```python
from build123d import *

# Parameters (mm, degrees)
PAD_DEPTH     = 1
SKETCH001_R   = 5.125
SKETCH001_R_2 = 9.9
PAD001_DEPTH  = 1
FILLET_R      = 1


with BuildPart() as part:
    # Sketch → Pad (new body)
    with BuildSketch(Plane.XY):
        with BuildLine():
            Line((70.272578, 45.492899), (78.436266, 3.274963))
            ThreePointArc((46.573742, -8.646925), (67.545071, -16.156101), (78.436266, 3.274963))
            Line((36.055693, 9.509252), (46.573742, -8.646925))
            ThreePointArc((5.490533, 14.509252), (19.215175, 2.485526), (36.055693, 9.509252))
            Line((-5.490533, 14.509252), (5.490533, 14.509252))
            ThreePointArc((-36.055693, 9.509252), (-19.215175, 2.485526), (-5.490533, 14.509252))
            Line((-46.573742, -8.646925), (-36.055693, 9.509252))
            ThreePointArc((-78.436265, 3.274968), (-67.545074, -16.1561), (-46.573742, -8.646925))
            Line((-70.272577, 45.492905), (-78.436265, 3.274968))
            ThreePointArc((-59.5, 62.051362), (-66.503327, 54.824144), (-70.272577, 45.492905))
            Line((-59.5, 62.051362), (-56.5, 72.051362))
            ThreePointArc((-32.5, 72.051362), (-44.5, 76.759252), (-56.5, 72.051362))
            Line((-32.5, 72.051362), (-30.237367, 64.509252))
            Line((-30.237367, 64.509252), (30.237367, 64.509252))
            Line((30.237367, 64.509252), (32.5, 72.051362))
            ThreePointArc((56.5, 72.051362), (44.5, 76.759252), (32.5, 72.051362))
            Line((56.5, 72.051362), (59.5, 62.051362))
            ThreePointArc((70.272578, 45.492899), (66.503328, 54.824142), (59.5, 62.051362))
        make_face()
    extrude(amount=PAD_DEPTH)

    # Sketch001 (on Face20 of Pad) → Pad001 (join)
    with BuildSketch(Plane.XY.offset(1)):
        with BuildLine():
            ThreePointArc((-59.5, 62.051362), (-66.503327, 54.824144), (-70.272577, 45.492905))
            Line((-70.272577, 45.492905), (-78.436265, 3.274968))
            ThreePointArc((-78.436265, 3.274968), (-67.545074, -16.1561), (-46.573742, -8.646925))
            Line((-46.573742, -8.646925), (-36.055693, 9.509252))
            ThreePointArc((-36.055693, 9.509252), (-19.215175, 2.485526), (-5.490533, 14.509252))
            Line((-5.490533, 14.509252), (5.490533, 14.509252))
            ThreePointArc((5.490533, 14.509252), (19.215175, 2.485526), (36.055693, 9.509252))
            Line((36.055693, 9.509252), (46.573742, -8.646925))
            ThreePointArc((46.573742, -8.646925), (67.545071, -16.156101), (78.436266, 3.274963))
            Line((78.436266, 3.274963), (70.272578, 45.492899))
            ThreePointArc((70.272578, 45.492899), (66.503328, 54.824142), (59.5, 62.051362))
            Line((59.5, 62.051362), (56.5, 72.051362))
            ThreePointArc((56.5, 72.051362), (44.5, 76.759252), (32.5, 72.051362))
            Line((32.5, 72.051362), (30.237367, 64.509252))
            Line((30.237367, 64.509252), (-30.237367, 64.509252))
            Line((-30.237367, 64.509252), (-32.5, 72.051362))
            ThreePointArc((-32.5, 72.051362), (-44.5, 76.759252), (-56.5, 72.051362))
            Line((-56.5, 72.051362), (-59.5, 62.051362))
        make_face()
        with BuildLine():
            ThreePointArc((55.140028, 70.584912), (44.5, 74.759252), (33.859972, 70.584912))
            Line((31.437274, 62.509252), (33.859972, 70.584912))
            Line((-31.437274, 62.509252), (31.437274, 62.509252))
            Line((-31.437274, 62.509252), (-33.859972, 70.584912))
            ThreePointArc((-33.859972, 70.584912), (-44.5, 74.759252), (-55.140028, 70.584912))
            Line((-58.357143, 60.410059), (-55.140028, 70.584912))
            ThreePointArc((-58.357143, 60.410059), (-64.826883, 53.733485), (-68.308952, 45.113198))
            Line((-76.47264, 2.895262), (-68.308952, 45.113198))
            ThreePointArc((-76.47264, 2.895262), (-66.844196, -14.282929), (-48.304323, -7.644383))
            Line((-48.304323, -7.644383), (-36.03269, 13.538817))
            ThreePointArc((-36.03269, 13.538817), (-35.306977, 12.060301), (-34.426047, 10.668673))
            ThreePointArc((-34.426047, 10.668673), (-19.538053, 4.459292), (-7.404674, 15.088962))
            ThreePointArc((-7.404674, 15.088962), (-7.209276, 15.794824), (-7.047993, 16.509252))
            Line((-7.047993, 16.509252), (7.047993, 16.509252))
            ThreePointArc((7.047993, 16.509252), (7.209276, 15.794824), (7.404674, 15.088962))
            ThreePointArc((7.404674, 15.088962), (19.538053, 4.459292), (34.426047, 10.668673))
            ThreePointArc((34.426047, 10.668673), (35.306977, 12.060301), (36.03269, 13.538817))
            Line((48.304323, -7.644383), (36.03269, 13.538817))
            ThreePointArc((48.304323, -7.644383), (66.844194, -14.28293), (76.472641, 2.895257))
            Line((76.472641, 2.895257), (68.308953, 45.113193))
            ThreePointArc((68.308953, 45.113193), (64.826884, 53.733483), (58.357143, 60.410059))
            Line((55.140028, 70.584912), (58.357143, 60.410059))
        make_face(mode=Mode.SUBTRACT)
        with Locations((30.375, 40.509252)):
            Circle(SKETCH001_R)
        with Locations((44.5, 54.634252)):
            Circle(SKETCH001_R)
        with Locations((58.625, 40.509252)):
            Circle(SKETCH001_R)
        with Locations((44.5, 26.384252)):
            Circle(SKETCH001_R)
        with Locations((-22, 19.509252)):
            Circle(SKETCH001_R_2)
        with Locations((22, 19.509252)):
            Circle(SKETCH001_R_2)
        Polygon((-58.4, 36.709252), (-51.8, 36.709252), (-49.55, 39.509252), (-49.55, 41.509252), (-51.8, 44.309252), (-58.4, 44.309252), align=None)
        Polygon((-40.7, 26.609252), (-48.3, 26.609252), (-48.3, 33.209252), (-45.5, 35.459252), (-43.5, 35.459252), (-40.7, 33.209252), align=None)
        Polygon((-30.6, 44.309252), (-37.2, 44.309252), (-39.45, 41.509252), (-39.45, 39.509252), (-37.2, 36.709252), (-30.6, 36.709252), align=None)
        Polygon((-48.3, 54.409252), (-40.7, 54.409252), (-40.7, 47.809252), (-43.5, 45.559252), (-45.5, 45.559252), (-48.3, 47.809252), align=None)
    extrude(amount=PAD001_DEPTH)

    # Fillet
    fillet_edges = [part.edges().sort_by_distance(p)[0] for p in [
        (-36.03269, 13.538817, 1.5),
        (-48.3, 26.609252, 1.5),
        (-58.4, 36.709252, 1.5),
        (-58.4, 44.309252, 1.5),
        (-48.3, 54.409252, 1.5),
        (-31.437274, 62.509252, 1.5),
        (-40.7, 54.409252, 1.5),
        (-30.6, 44.309252, 1.5),
        (-30.6, 36.709252, 1.5),
        (-40.7, 26.609252, 1.5),
        (-7.047993, 16.509252, 1.5),
        (36.03269, 13.538817, 1.5),
        (31.437274, 62.509252, 1.5),
        (58.357143, 60.410059, 1.5),
        (7.047993, 16.509252, 1.5),
        (-58.357143, 60.410059, 1.5),
        (-37.2, 36.709252, 1.5),
        (-39.45, 39.509252, 1.5),
        (-43.5, 45.559252, 1.5),
        (-45.5, 45.559252, 1.5),
        (-48.3, 47.809252, 1.5),
        (-51.8, 36.709252, 1.5),
        (-48.3, 33.209252, 1.5),
        (-51.8, 44.309252, 1.5),
        (-49.55, 41.509252, 1.5),
        (-49.55, 39.509252, 1.5),
        (-45.5, 35.459252, 1.5),
        (-43.5, 35.459252, 1.5),
        (-40.7, 33.209252, 1.5),
        (-37.2, 44.309252, 1.5),
        (-40.7, 47.809252, 1.5),
        (-39.45, 41.509252, 1.5),
    ]]
    fillet(fillet_edges, radius=FILLET_R)


solid = part.part
```
Source: CAD feature listing. Evaluate the final solid. Frame: model axes, mm. A direction names the side the tool comes from. Give positions to 0.01 mm unless a question says otherwise; leave off trailing zeros. Loops run counter-clockwise (first coordinate to the right, second up) from the corner with the lowest first, then second, coordinate; pieces in that order, holes last. Notation, with made-up numbers: (-4, 0) -> (46, 0) arc R18 cw to (46, 13) -> close; hole circle Ø3 at (28.5, 48). An arc over 180 degrees is marked (long way). Use a Markdown table: item, result. Add a question column.
(1) Section query C-C (z = 0.65). Output: boundary loops of the cut face in (x, y), then the cut area to 3 significant figures.
(2) Ray query, line 1 (X direction, y = 19, z = 1.2); line 2 (Y direction, x = -15, z = 1.95); line 3 (Y direction, x = 60, z = 1.5). Return the intervals inside material, ascending.
(3) Pull-direction query (Y, two-part tool) for faces 3 (the face through (42.71, 2.01, 1.49)), 4 (the face through (-66.426, 54.943, 0.986)), 5 (the face through (18.95, 2.53, 0.99)); classes: +Y half, -Y half, draft (parallel to the pull), parting line (faces both ways), or undercut.
(4) Section query D-D (y = 58). Output: boundary loops of the cut face in (x, z), then the cut area to 3 significant figures.
(5) First-contact query: pin 1 Ø0.5 at (y, z) = (40.5, 1.5) entering from +X; pin 2 Ø1.1 at (y, z) = (39.5, 1.5) entering from -X; pin 3 Ø1.5 at (x, y) = (-60.5, 22) entering from -Z; pin 4 Ø0.6 at (x, z) = (-0.5, 0.5) entering from -Y. Flat tips, straight axial feed; report the tip coordinate or a pass-through.
(6) Section query B-B (x = -22). Output: boundary loops of the cut face in (y, z), then the cut area to 4 significant figures.
(7) Access query for faces 1 (the face through (-57.98, 67.12, 0.99)), 2 (the face through (31.145, 15.717, 1.493)). Directions: +Z, -Z, +X, -X, +Y, -Y. A direction counts if a zero-diameter tool reaches every point of the face in a straight line with its end or side. Return the directions, or none.
(8) Section query A-A (y = -10.5). Output: boundary loops of the cut face in (x, z), then the cut area to 3 significant figures.
Checked values:
| question | item | result |
|---|---|---|
| 1 | outline | (-78.44, 3.27) arc R17.25 ccw to (-46.57, -8.65) -> (-36.06, 9.51) arc R17.25 ccw to (-5.49, 14.51) -> (5.49, 14.51) arc R17.25 ccw to (36.06, 9.51) -> (46.57, -8.65) arc R17.25 ccw to (78.44, 3.27) -> (70.27, 45.49) arc R26.25 ccw to (59.5, 62.05) -> (56.5, 72.05) arc R17.65 ccw to (32.5, 72.05) -> (30.24, 64.51) -> (-30.24, 64.51) -> (-32.5, 72.05) arc R17.65 ccw to (-56.5, 72.05) -> (-59.5, 62.05) arc R26.25 ccw to (-70.27, 45.49) -> close |
| 1 | area | 10,300 mm^2 |
| 2 | line 1 | -75.4 to -73.36, -31.89 to -12.11, 12.11 to 31.89, 73.36 to 75.4 |
| 2 | line 2 | 3.74 to 5.96, 12.51 to 26.51, 62.51 to 64.51 |
| 2 | line 3 | -17.18 to -15.18, 35.57 to 45.45, 59.16 to 61.69 |
| 3 | face 3 | undercut |
| 3 | face 4 | +Y half |
| 3 | face 5 | -Y half |
| 4 | outline | (-64.07, 0) -> (64.07, 0) -> (64.07, 2) -> (61.3, 2) -> (61.3, 1) -> (48.36, 1) -> (48.36, 2) -> (40.64, 2) -> (40.64, 1) -> (-61.3, 1) -> (-61.3, 2) -> (-64.07, 2) -> close |
| 4 | area | 141 mm^2 |
| 5 | pin 1 | x = 71.29 |
| 5 | pin 2 | x = -71.54 |
| 5 | pin 3 | z = 0 |
| 5 | pin 4 | y = 14.51 |
| 6 | outline | (2.26, 0) -> (64.51, 0) -> (64.51, 2) -> (62.51, 2) -> (62.51, 1) -> (29.41, 1) -> (29.41, 2) -> (9.61, 2) -> (9.61, 1) -> (4.26, 1) -> (4.26, 2) -> (2.26, 2) -> close |
| 6 | area | 86.05 mm^2 |
| 7 | face 1 | +Z, -Z, -X, +Y |
| 7 | face 2 | +Z |
| 8 | outline | (-75.19, 0) -> (-47.81, 0) -> (-47.81, 2) -> (-50.44, 2) -> (-50.44, 1) -> (-72.56, 1) -> (-72.56, 2) -> (-75.19, 2) -> close; (47.81, 0) -> (75.19, 0) -> (75.19, 2) -> (72.56, 2) -> (72.56, 1) -> (50.44, 1) -> (50.44, 2) -> (47.81, 2) -> close |
| 8 | area | 65.3 mm^2 |
